```python
from build123d import *

# Parameters (mm, degrees)
SKETCH2_W           = 1500
SKETCH2_H           = 1500
BOSS_EXTRUDE1_DEPTH = 10
BOSS_EXTRUDE2_DEPTH = 110
BOSS_EXTRUDE3_DEPTH = 110


with BuildPart() as part:
    # Sketch2 → Boss-Extrude1 (new body)
    with BuildSketch(Plane(origin=(0, 0, 0), x_dir=(1, 0, 0), z_dir=(0, 1, 0))):
        Rectangle(SKETCH2_W, SKETCH2_H)
    extrude(amount=BOSS_EXTRUDE1_DEPTH)

    # Sketch3 → Boss-Extrude2 (add)
    with BuildSketch(Plane(origin=(0, 10, 0), x_dir=(1, 0, 0), z_dir=(0, 1, 0))):
        with BuildLine():
            ThreePointArc((750, -600), (-204.594154602, -204.594154602), (-600, 750))
            Line((-600, 750), (-620, 750))
            ThreePointArc((-620, 750), (-218.736290226, -218.736290226), (750, -620))
            Line((750, -620), (750, -600))
        make_face()
        with BuildLine():
            Line((620, 750), (600, 750))
            ThreePointArc((600, 750), (643.933982822, 643.933982822), (750, 600))
            Line((750, 600), (750, 620))
            ThreePointArc((750, 620), (658.076118446, 658.076118446), (620, 750))
        make_face()
    extrude(amount=BOSS_EXTRUDE2_DEPTH)

    # Sketch4 → Boss-Extrude3 (add)
    with BuildSketch(Plane(origin=(0, 10, 0), x_dir=(1, 0, 0), z_dir=(0, 1, 0))):
        with BuildLine():
            ThreePointArc((269.66991411, 219.66991411), (265.863890736, 238.804085728), (255.025253169, 255.025253169))
            Line((255.025253169, 255.025253169), (184.314575051, 184.314575051))
            ThreePointArc((184.314575051, 184.314575051), (238.804085728, 173.475937485), (269.66991411, 219.66991411))
        make_face()
        with BuildLine():
            Line((184.314575051, 184.314575051), (255.025253169, 255.025253169))
            ThreePointArc((255.025253169, 255.025253169), (184.314575051, 255.025253169), (184.314575051, 184.314575051))
        make_face()
    extrude(amount=BOSS_EXTRUDE3_DEPTH)


solid = part.part
```
Here's how the part is built. I have some questions about the finished solid (model axes, mm). A direction names the side the tool comes from. Give positions to 0.01 mm unless a question says otherwise; leave off trailing zeros. Order: outer loops, then holes, each group sorted by start corner. A loop starts at its lowest first (then second) coordinate and runs counter-clockwise, first axis right, second up. Notation, with made-up numbers: (44, 79.5) -> (100, 79.5) arc R20 cw to (100, 91.5) -> close; hole circle Ø7 at (50, -10.75). An arc over 180 degrees is marked (long way). Use CSV: the item, a comma, the result in double quotes. Start each with the question number.
Item 1: Suppose I cut it at B-B (x = -9.5). List the corners of the cut face in (y, z) for me.
Item 2: Suppose I cut it at A-A (y = 48.5). List the corners of the cut face in (x, z) for me.
Item 3: If I drill on probe 1 along Y at (x, z) = (-118.5, 332); probe 2 along X at (y, z) = (107.5, -187); probe 3 along X at (y, z) = (49.5, -490), over which ranges is the centre line in solid material (lowest first)? Write a range as [from, to].
Item 4: Thinking about a two-plate mould opening in Z: for faces 6 (the cylindrical face through (642.77, 64.23, -645.11)), 7 (the flat face through (750, 2, 4)), 8 (the cylindrical face through (-229.329, 64.23, 208.026)), which applies, pulls with the +Z half, pulls with the -Z half, needs draft (parallel to the pull), parting line crosses it, or undercut?
Item 5: On a 3-axis mill with a long thin cutter (end or side, diameter ignored), from which of +Z, -Z, +X, -X, +Y, -Y can I reach the whole of each face in a straight line? I mean faces 1 (the flat face through (-337, 10, 274)), 2 (the flat face through (-293, 120, 135)), 3 (the cylindrical face through (659.092, 64.23, -657.071)), 4 (the flat face through (-10, 0, -10)), 5 (the flat face through (66, 10, -234)). Say none if no direction works.
Item 6: I'm going to push flat-ended pins straight in: P1, Ø3, axis at x = -283, y = 55, coming from the +Z side; P2, Ø6, axis at x = -353, z = 448, coming from the -Y side; P3, Ø12, axis at x = -234, y = 51.5, coming from the -Z side; P4, Ø6, axis at y = 36.5, z = 227.5, coming from the -X side. Where does each tip first touch, or does it pass through?
Item 7: Suppose I cut it at C-C (z = 45). List the corners of the cut face in (x, y) for me.
Item 8: Suppose I cut it at D-D (z = 642.5). List the corners of the cut face in (x, y) for me.
Answer block:
1,outline,"(0, -750) -> (10, -750) -> (10, 366.09) -> (120, 366.09) -> (120, 390.2) -> (10, 390.2) -> (10, 750) -> (0, 750) -> close"
2,outline,"(-620, -750) -> (-600, -750) arc R1350 cw to (750, 600) -> (750, 620) arc R1370 ccw to start; circle Ø100 at (219.67, -219.67); (600, -750) -> (620, -750) arc R130 cw to (750, -620) -> (750, -600) arc R150 ccw to start"
3,probe 1,"y = [0, 10]"
3,probe 2,"x = [-498.97, -477], [181.82, 257.52]"
3,probe 3,"x = [-595.1, -574.73]"
4,face 6,"undercut"
4,face 7,"needs draft"
4,face 8,"pulls with the +Z half"
5,face 1,"+Z, -X, +Y"
5,face 2,"+Z, -Z, +X, -X, +Y"
5,face 3,"-Z, +X, +Y"
5,face 4,"+Z, -Z, +X, -X, -Y"
5,face 5,"+Y"
6,P1,"stops at z = 151.61"
6,P2,"stops at y = 0"
6,P3,"stops at z = 167.82"
6,P4,"stops at x = -212.94"
7,outline,"(-750, 0) -> (750, 0) -> (750, 10) -> (-341.09, 10) -> (-341.09, 120) -> (-365.74, 120) -> (-365.74, 10) -> (-750, 10) -> close"
8,outline,"(-750, 0) -> (750, 0) -> (750, 10) -> (-750, 10) -> close"
